Can you work these out from the drawing? Everything is in mm from the part's minimum corner. Coordinates: 2 decimals unless noted, no trailing zeros. Order: outer loops, then holes, each group sorted by start corner. A loop starts at its lowest first (then second) coordinate and runs counter-clockwise, first axis right, second up. Notation, with made-up numbers: (15.25, 24) - (19.25, 24) arc R20 ccw to (19.25, 46) - close; hole circle Ø1 at (-10, 89.5). An arc over 180 degrees is marked (long way). Use a Markdown table: item, result. Add a question column.
(1) If I drill on L1, parallel to Y at x = 12, z = 3; L2, parallel to Y at x = 11.25, z = 4.25; L3, parallel to X at y = 10, z = 7.5, over which ranges is the centre line in solid material (lowest first)? Write a range as [from, to].
(2) I want a section at C-C (y = 11). List the corners of the cut face in (x, z) for me, and give its area (3 significant figures).
(3) I want a section at B-B (z = 9.5). List the corners of the cut face in (x, y) for me, and give its area (3 significant figures).
(4) For pin 1 Ø2 at (x, y) = (9, 11.5) entering from -Z; pin 2 Ø3.5 at (x, y) = (12, 5) entering from +Z, each with a flat end and sliding along its axis, tell me the tip position at first contact or that it passes through.
(5) We'd pull the mould along X, two halves only. Please class the marked faces 1, 2 and 3: pulls with the +X half, pulls with the -X half, needs draft (parallel to the pull), parting line crosses it, or undercut.
(6) I want a section at D-D (y = 5.75). List the corners of the cut face in (x, z) for me.
(7) I want a section at A-A (x = 19). List the corners of the cut face in (y, z) for me.
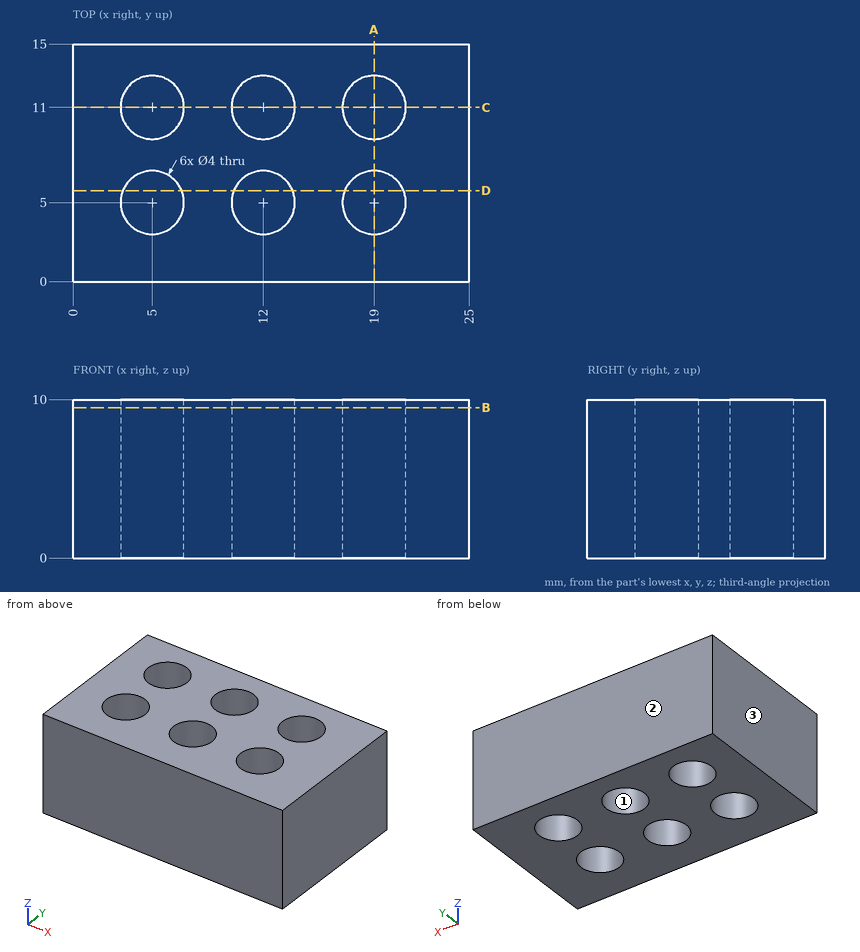
Answers follow:
| question | item | result |
|---|---|---|
| 1 | L1 | y = [0, 3], [7, 9], [13, 15] |
| 1 | L2 | y = [0, 3.15], [6.85, 9.15], [12.85, 15] |
| 1 | L3 | x = [0, 3.27], [6.73, 10.27], [13.73, 17.27], [20.73, 25] |
| 2 | outline | (0, 0) - (3, 0) - (3, 10) - (0, 10) - close; (7, 0) - (10, 0) - (10, 10) - (7, 10) - close; (14, 0) - (17, 0) - (17, 10) - (14, 10) - close; (21, 0) - (25, 0) - (25, 10) - (21, 10) - close |
| 2 | area | 130 mm² |
| 3 | outline | (0, 0) - (25, 0) - (25, 15) - (0, 15) - close; hole circle Ø4 at (5, 5); hole circle Ø4 at (5, 11); hole circle Ø4 at (12, 5); hole circle Ø4 at (12, 11); hole circle Ø4 at (19, 5); hole circle Ø4 at (19, 11) |
| 3 | area | 300 mm² |
| 4 | pin 1 | stops at z = 0 |
| 4 | pin 2 | passes through |
| 5 | face 1 | undercut |
| 5 | face 2 | needs draft |
| 5 | face 3 | pulls with the -X half |
| 6 | outline | (0, 0) - (3.15, 0) - (3.15, 10) - (0, 10) - close; (6.85, 0) - (10.15, 0) - (10.15, 10) - (6.85, 10) - close; (13.85, 0) - (17.15, 0) - (17.15, 10) - (13.85, 10) - close; (20.85, 0) - (25, 0) - (25, 10) - (20.85, 10) - close |
| 7 | outline | (0, 0) - (3, 0) - (3, 10) - (0, 10) - close; (7, 0) - (9, 0) - (9, 10) - (7, 10) - close; (13, 0) - (15, 0) - (15, 10) - (13, 10) - close |
